from build123d import *

# Parameters (mm, degrees)
SKETCH1_R           = 1.5
BOSS_EXTRUDE1_DEPTH = 30


with BuildPart() as part:
    # Sketch1 → Boss-Extrude1 (new, symmetric)
    with BuildSketch(Plane(origin=(0, 0, 0), x_dir=(1, 0, 0), z_dir=(0, 1, 0))):
        with Locations(Location((0, 0, 0), (0, 0, 270))):
            Circle(SKETCH1_R)
    extrude(amount=BOSS_EXTRUDE1_DEPTH, both=True)

    # Sketch2 → Revolve1 (revolve)
    with BuildSketch(Plane.XY):
        with BuildLine():
            Line((0, 30), (-1.731543481, 30))
            ThreePointArc((-1.731543481, 30), (-1.825836483, 30.066700905), (-1.794340914, 30.177823405))
            add(Edge.make_bspline(
                [(-1.794340914, 30.177823405), (-1.296972614, 30.579160925), (-0.657911989, 31), (0, 31)],
                knots=[0, 0, 0, 0, 1, 1, 1, 1], degree=3))
            Line((0, 31), (0, 30))
        make_face()
    revolve1 = revolve(axis=Axis((0, 31, 0), (0, -1, 0)))

    # Mirror1: Revolve1 across plane
    add(revolve1.mirror(Plane.ZX))


solid = part.part
Read the model definition and answer for the solid it produces. Units are mm, in the model's axes. Coordinates: 2 decimals unless noted, no trailing zeros. Order: outer loops, then holes, each group sorted by start corner. A loop starts at its lowest first (then second) coordinate and runs counter-clockwise, first axis right, second up. Notation, with made-up numbers: (-31.5, 33.5) - (-20.5, 33.5) arc R20 cw to (-20.5, 61.5) - close; hole circle Ø4 at (-14.75, -30.75). An arc over 180 degrees is marked (long way). Use one line per item in the form item = value.
(1) Given pin 1 Ø1.5 at (y, z) = (12, 1) entering from +X; pin 2 Ø2 at (x, y) = (0.5, -24) entering from -Z; pin 3 Ø1.5 at (x, z) = (-1, -1) entering from +Y, each flat-ended and moving along its own axis, determine where each tip first touches the part or whether it passes through.
Computed values:
pin_1 = 1.48
pin_2 = -1.5
pin_3 = 30.87
(2) Straight lines are drawn through the part: L1, parallel to X at y = 19, z = 0.2; L2, parallel to Y at x = 0.3, z = -1.55; L3, parallel to Y at x = -1.65, z = 0.45. For each, find the intervals that lie inside material, in ascending order.
Computed values:
L1 = -1.49 to 1.49
L2 = -30.35 to -30, 30 to 30.35
L3 = -30.24 to -30, 30 to 30.24
(3) Section A-A, the plane y = 7.5 is taken. Give the vertices of the cut face in (x, z), then the cut area to 3 significant figures.
Computed values:
outline = circle Ø3 at (0, 0)
area = 7.07 mm²
